Build history of the part. All positions in model axes, mm. Give positions to 0.01 mm unless a question says otherwise; leave off trailing zeros. Loops run counter-clockwise (first coordinate to the right, second up) from the corner with the lowest first, then second, coordinate; pieces in that order, holes last. Notation, with made-up numbers: (68.25, -8.75) -> (94.25, -8.75) arc R31 ccw to (94.25, 27.25) -> close; hole circle Ø5 at (-24.5, -16.5). An arc over 180 degrees is marked (long way). Answer in a Markdown table with one row per item. Add a question column.
Autodesk Inventor part; units mm, degrees
ref_plane "YZ Plane" through (0, 0, 0) normal (1, 0, 0) x (0, 1, 0)
ref_plane "XZ Plane" through (0, 0, 0) normal (0, 1, 0) x (-1, 0, 0)
ref_plane "XY Plane" through (0, 0, 0) normal (0, 0, 1) x (1, 0, 0)
sketch "Sketch2" plane through (0, 0, 0) normal (0, 0, 1) x (1, 0, 0)
  line L0 (0, 0) -> (300.1103, 0)
  line L1 (300.1103, 0) -> (300.1103, 100.8009)
  line L2 (300.1103, 100.8009) -> (0, 100.8009)
  line L3 (0, 100.8009) -> (0, 0)
  circle A0 centre (10, 90.343) radius 5.4183
  circle A1 centre (10, 10) radius 5.4183
  circle A2 centre (289.5422, 90.6602) radius 5.4183
  circle A3 centre (290.3474, 9.1425) radius 5.4183
  spline S0 degree 3 poles (47.0614, 25.4545) (47.528, 43.4805) (54.12, 78.9822) (64.9978, 83.5345) knots 0 0 0 0 1 1 1 1
  spline S1 degree 3 poles (64.9978, 83.5345) (83.6065, 81.6461) (82.7385, 43.7232) (85.9237, 25.4545) knots 0 0 0 0 1 1 1 1
  spline S2 degree 1 poles (55.389, 24.3869) (57.7378, 50.4375) knots 0 0 1 1
  spline S3 degree 2 poles (47.0614, 25.4545) (49.1255, 15.705) (55.389, 24.3869) knots 0 0 0 1 1 1
  spline S4 degree 1 poles (78.8772, 24.3869) (74.3931, 50.651) knots 0 0 1 1
  spline S5 degree 2 poles (78.8772, 24.3869) (83.5505, 13.6282) (85.9237, 25.4545) knots 0 0 0 1 1 1
  spline S6 degree 4 poles (59.019, 57.911) (58.4576, 61.6443) (68.1339, 91.1213) (71.7472, 59.0435) (72.6849, 58.1245) knots 0 0 0 0 0 1 1 1 1 1
  spline S7 degree 1 poles (96.1731, 25.0275) (96.1731, 55.7757) knots 0 0 1 1
  spline S8 degree 1 poles (103.4331, 25.0275) (103.4331, 44.0316) knots 0 0 1 1
  spline S9 degree 2 poles (103.4331, 44.0316) (109.8398, 52.1437) (116.2448, 44.0316) knots 0 0 0 1 1 1
  spline S10 degree 2 poles (103.4331, 52.3592) (109.9746, 59.5015) (116.2448, 51.7186) knots 0 0 0 1 1 1
  spline S11 degree 1 poles (103.4331, 52.3592) (103.4331, 55.7757) knots 0 0 1 1
  spline S12 degree 2 poles (103.4331, 55.7757) (100.4586, 63.4655) (96.1731, 55.7757) knots 0 0 0 1 1 1
  spline S13 degree 2 poles (116.2448, 51.7186) (121.8944, 46.0101) (116.2448, 44.0316) knots 0 0 0 1 1 1
  spline S14 degree 2 poles (96.1731, 25.0275) (100.5122, 14.8704) (103.4331, 25.0275) knots 0 0 0 1 1 1
  spline S15 degree 1 poles (137.5551, 24.3869) (137.5551, 48.0887) knots 0 0 1 1
  line L4 (144.815, 24.3869) -> (144.815, 48.0887)
  line L5 (144.815, 48.0887) -> (152.5021, 48.0887)
  line L6 (137.5551, 48.0887) -> (129.868, 48.0887)
  line L7 (137.5551, 55.7757) -> (129.868, 55.7757)
  line L8 (152.5021, 55.7757) -> (144.815, 55.7757)
  line L9 (144.815, 55.7757) -> (144.815, 69.6551)
  line L10 (137.5551, 55.7757) -> (137.5551, 69.6551)
  spline S16 degree 2 poles (137.5551, 24.3869) (140.9704, 16.0905) (144.815, 24.3869) knots 0 0 0 1 1 1
  spline S17 degree 2 poles (137.5551, 69.6551) (140.8285, 77.0951) (144.815, 69.6551) knots 0 0 0 1 1 1
  spline S18 degree 2 poles (152.5021, 55.7757) (161.0322, 52.5769) (152.5021, 48.0887) knots 0 0 0 1 1 1
  spline S19 degree 2 poles (129.868, 55.7757) (117.4806, 52.6672) (129.868, 48.0887) knots 0 0 0 1 1 1
  spline S20 degree 2 poles (165.9544, 27.1628) (181.1135, 4.9444) (193.2862, 27.1628) knots 0 0 0 1 1 1
  spline S21 degree 1 poles (165.9544, 27.1628) (165.9544, 52.359) knots 0 0 1 1
  spline S22 degree 1 poles (172.7874, 52.359) (172.7874, 30.1522) knots 0 0 1 1
  spline S23 degree 2 poles (172.7874, 30.1522) (181.8365, 16.2304) (186.8803, 29.7251) knots 0 0 0 1 1 1
  spline S24 degree 1 poles (186.8803, 29.7251) (186.5322, 52.344) knots 0 0 1 1
  spline S25 degree 1 poles (193.2862, 27.1628) (194.0062, 52.359) knots 0 0 1 1
  spline S26 degree 2 poles (165.9544, 52.359) (167.9027, 63.2961) (172.7874, 52.359) knots 0 0 0 1 1 1
  spline S27 degree 2 poles (194.0062, 52.359) (189.5472, 63.0062) (186.5322, 52.344) knots 0 0 0 1 1 1
  line L11 (200.8451, 22.6644) -> (200.8451, 58.3238)
  line L12 (207.6781, 22.6644) -> (207.6781, 43.3768)
  spline S28 degree 2 poles (200.8451, 22.6644) (204.6115, 13.7645) (207.6781, 22.6644) knots 0 0 0 1 1 1
  spline S29 degree 2 poles (207.6781, 43.3768) (215.6878, 50.9193) (222.6251, 43.3768) knots 0 0 0 1 1 1
  spline S30 degree 2 poles (207.6781, 51.7044) (215.1483, 58.6179) (222.6251, 52.9856) knots 0 0 0 1 1 1
  spline S31 degree 1 poles (207.6781, 51.7044) (207.6781, 58.3238) knots 0 0 1 1
  spline S32 degree 2 poles (200.8451, 58.3238) (204.6164, 65.9043) (207.6781, 58.3238) knots 0 0 0 1 1 1
  spline S33 degree 2 poles (222.6251, 52.9856) (229.0495, 47.1979) (222.6251, 43.3768) knots 0 0 0 1 1 1
  spline S34 degree 1 poles (59.019, 57.911) (67.7644, 58.3238) knots 0 0 1 1
  spline S35 degree 1 poles (57.7378, 50.4375) (66.4498, 51.7044) knots 0 0 1 1
  spline S36 degree 1 poles (72.6849, 58.1245) (74.3931, 50.651) knots 0 0 1 1
  spline S37 degree 2 poles (67.7644, 58.3238) (73.9281, 55.5594) (66.4498, 51.7044) knots 0 0 0 1 1 1
  spline S38 degree 3 poles (250.3077, 16.0597) (229.6641, 17.286) (235.0288, 49.9642) (248.7928, 59.6179) knots 0 0 0 0 1 1 1 1
  spline S39 degree 4 poles (250.3077, 16.0597) (265.1319, 9.4554) (277.4389, 34.9714) (273.4781, 48.5926) (254.3403, 65.288) (256.1147, 50.4005) knots 0 0 0 0 0 0.544263 1 1 1 1 1
  spline S40 degree 3 poles (248.7928, 50.4005) (245.7595, 44.1304) (238.6673, 17.9358) (259.1445, 24.3869) knots 0 0 0 0 1 1 1 1
  spline S41 degree 2 poles (259.1445, 24.3869) (271.6388, 36.6081) (256.1147, 50.4005) knots 0 0 0 1 1 1
  spline S42 degree 2 poles (248.7928, 59.6179) (255.8815, 56.0643) (248.7928, 50.4005) knots 0 0 0 1 1 1
  point P0 (50.0508, 50.4375)
  point P1 (57.7364, 75.2009)
  point P2 (76.3178, 75.1435)
  point P3 (82.9341, 50.4375)
  point P4 (50.0483, 20.3336)
  point P5 (82.9302, 19.2685)
  point P6 (62.1793, 68.1604)
  point P7 (66.4499, 71.5768)
  point P8 (70.5496, 65.8115)
  point P9 (109.8396, 48.0876)
  point P10 (109.8361, 55.7733)
  point P11 (100.2313, 59.6176)
  point P12 (119.033, 46.517)
  point P13 (100.2294, 19.9509)
  point P14 (141.048, 20.239)
  point P15 (140.9494, 73.3742)
  point P16 (156.7647, 52.3472)
  point P17 (123.6758, 52.3588)
  point P18 (180.6877, 16.0597)
  point P19 (181.2472, 23.0958)
  point P20 (168.5193, 57.821)
  point P21 (189.8394, 57.6769)
  point P22 (204.4763, 18.215)
  point P23 (215.5971, 47.1459)
  point P24 (215.3469, 55.4961)
  point P25 (204.4901, 62.1132)
  point P26 (225.828, 47.4324)
  point P27 (70.5492, 55.5893)
  point P28 (238.1887, 24.3868)
  point P29 (238.1887, 43.3767)
  point P30 (267.4763, 20.3332)
  point P31 (272.021, 36.2378)
  point P32 (267.4763, 50.4005)
  point P33 (259.1445, 58.3238)
  point P34 (245.763, 40.4941)
  point P35 (246.5206, 27.1626)
  point P36 (264.6991, 36.2378)
  point P37 (252.3275, 55.7757)
  dimension "d0" = 100.8009
  dimension "d1" = 300.1103
  dimension "d3" = 10.8366
  dimension "d4" = 10.8366
  dimension "d5" = 10.8366
  dimension "d6" = 10.8366
  dimension "d26" = 7.6871
  dimension "d27" = 8.541
  dimension "d28" = 8.3276
  dimension "d29" = 7.26
  dimension "d30" = 7.474
  dimension "d31" = 6.8329
  dimension "d32" = 7.26
  dimension "d33" = 8.3276
  dimension "d34" = 6.8329
extrude "Plate5" add sketch "Sketch2" along normal blind 10
equation "\"BendReliefDepth\" = 0.5 * Thickness"
properties part number "Name"
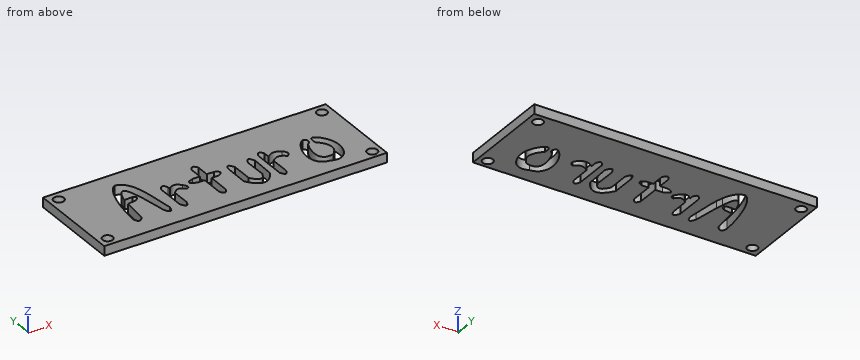
(1) Saw through at A-A, the plane x = 10. List the corners of the cut face in (y, z), then the cut area to 3 significant figures.
(2) Saw through at B-B, the plane y = 65. State how many separate pieces and enclosed holes the cut face has, then the cut area to 3 significant figures.
(3) Wall check: line 1 along Y through (x, z) = (10, 7); line 2 along X through (y, z) = (88, 9); line 3 along Y through (x, z) = (151.5, 8). Give the ranges that are in metal, low to high. Write a range as from..to.
(4) Flat gauge pin, fed straight in: pin 1 Ø8.5 at (x, y) = (10, 10) entering from -Z. Where does the tip first touch, or does it go through?
Worked answers:
| question | item | result |
|---|---|---|
| 1 | outline | (0, 0) -> (4.58, 0) -> (4.58, 10) -> (0, 10) -> close; (15.42, 0) -> (84.92, 0) -> (84.92, 10) -> (15.42, 10) -> close; (95.76, 0) -> (100.8, 0) -> (100.8, 10) -> (95.76, 10) -> close |
| 1 | area | 791 mm^2 |
| 2 | separate pieces | 4 |
| 2 | enclosed holes | 0 |
| 2 | area | 2,760 mm^2 |
| 3 | line 1 | 0..4.58, 15.42..84.92, 95.76..100.8 |
| 3 | line 2 | 0..5.11, 14.89..284.82, 294.26..300.11 |
| 3 | line 3 | 0..48.09, 55.78..100.8 |
| 4 | pin 1 | through |
